Input: part model. Units: mm. Frame: model coordinates. A direction names the side the tool comes from. Coordinates: 2 decimals unless noted, no trailing zeros. Write each loop counter-clockwise with the first axis right and the second up, starting at its lowest first coordinate (ties: lowest second). Pieces come first, ordered by that corner, then holes. Notation, with made-up numbers: M 73.25,69 L 114.25,69 A19 ccw 114.25,93 Z; hole C 25.5,-19.75 d6. An arc over 180 degrees is marked long. Write each question's results on one line, items separated by ' | '. Start each with the question number.
1. First-contact query: pin 1 (6.5 mm diameter, centred on x = -12.06, z = -5, fed in from +Y); pin 2 (3 mm diameter, centred on x = -12.06, z = -25, fed in from +Y); pin 3 (10 mm diameter, centred on x = -13, z = -14, fed in from +Y). Flat tips, straight axial feed; report the tip coordinate or a pass-through.
2. Section query B-B, the plane x = 0. Output: boundary loops of the cut face in (y, z).
3. Section query C-C, the plane y = 0. Output: boundary loops of the cut face in (x, z).
4. Pull-direction query (X, two-part tool) for faces 4 (the flat face through (16.961, -2, -15)), 5 (the flat face through (4, -5, -30)), 6 (the cylindrical face through (-1.08, -4.88, -14.79)); classes: +X half, -X half, draft (parallel to the pull), parting line (faces both ways), or undercut.
5. Set-up query: faces 1 (the flat face through (-13, 7.001, -15)), 2 (the flat face through (12, 7.001, -15)), 3 (the flat face through (0, 11.001, -15)). Return all of +Z, -Z, +X, -X, +Y, -Y with unobstructed straight access to the full face (end or side cutting, diameter ignored); none if empty.
6. Section query A-A, the plane z = -5. Output: boundary loops of the cut face in (x, y), and give its area (3 significant figures).
7. Ray query, probe 1 along X at (y, z) = (1.5, -26.25); probe 2 along Z at (x, y) = (11, 6.5); probe 3 along Y at (x, z) = (0, -13.25). Return the intervals inside material, ascending.
8. Section query D-D, the plane x = 10.5. Output: boundary loops of the cut face in (y, z).
```python
from build123d import *

# Parameters (mm, degrees)
BOSS_EXTRUDE2_DEPTH    = 30
HOLE_R                 = 5
CUT_EXTRUDE1_DEPTH     = 30
CUT_EXTRUDE2_START     = -10.999447078
CUT_EXTRUDE2_OUTLINE_R = 2
CUT_EXTRUDE2_DEPTH     = 17.999956595


# Read off the part's stored shape, not the designer's step: Cut-Extrude2
with BuildPart() as part:
    # body → Boss-Extrude2 (new body)
    with BuildSketch(Plane.XY):
        Polygon((-8.038514806, 7.000509517), (-5.875565247, 11.000552922), (5.877594601, 11.000552922), (8.04054416, 7.000509517), (16.961485195, 7.000509517), (16.961485195, -10.999447078), (-17.038514805, -10.999447078), (-17.038514805, 7.000509517), align=None)
    extrude(amount=-BOSS_EXTRUDE2_DEPTH)

    # hole → Cut-Extrude1 (cut)
    with BuildSketch(Plane.XY):
        Circle(HOLE_R)
    extrude(amount=-CUT_EXTRUDE1_DEPTH, mode=Mode.SUBTRACT)

    # Cut-Extrude2 outline → Cut-Extrude2 (cut)
    with BuildSketch(Plane(origin=(0, 0, 0), x_dir=(1, 0, 0), z_dir=(0, 1, 0)).offset(CUT_EXTRUDE2_START)):
        with Locations((-12.061902792, 5)):
            Circle(CUT_EXTRUDE2_OUTLINE_R)
        with Locations((-12.061902792, 24.999986325)):
            Circle(CUT_EXTRUDE2_OUTLINE_R)
        with Locations((11.938097208, 24.999986325)):
            Circle(CUT_EXTRUDE2_OUTLINE_R)
        with Locations((11.938097208, 5)):
            Circle(CUT_EXTRUDE2_OUTLINE_R)
    extrude(amount=CUT_EXTRUDE2_DEPTH, mode=Mode.SUBTRACT)


solid = part.part
```
Answer:
1) pin 1: y = 7 | pin 2: through | pin 3: y = 7.07
2) outline: M -11,-30 L -5,-30 L -5,0 L -11,0 Z; M 5,-30 L 11,-30 L 11,0 L 5,0 Z
3) outline: M -17.04,-30 L -5,-30 L -5,0 L -17.04,0 Z; M 5,-30 L 16.96,-30 L 16.96,0 L 5,0 Z; hole C -12.06,-25 d4; hole C -12.06,-5 d4; hole C 11.94,-25 d4; hole C 11.94,-5 d4
4) face 4: +X half | face 5: draft | face 6: undercut
5) face 1: +Z, -Z, -X, +Y | face 2: +Z, -Z, +X, +Y | face 3: +Z, -Z, +X, -X, +Y
6) outline: M -17.04,-11 L -14.06,-11 L -14.06,7 L -17.04,7 Z; M -10.06,-11 L 9.94,-11 L 9.94,7 L 8.04,7 L 5.88,11 L -5.88,11 L -8.04,7 L -10.06,7 Z; M 13.94,-11 L 16.96,-11 L 16.96,7 L 13.94,7 Z; hole C 0,0 d10 | area: 445 mm^2
7) probe 1: -17.04 to -13.62, -10.5 to -4.77, 4.77 to 10.38, 13.5 to 16.96 | probe 2: -30 to -26.77, -23.23 to -6.77, -3.23 to 0 | probe 3: -11 to -5, 5 to 11
8) outline: M -11,-30 L 7,-30 L 7,-26.39 L -11,-26.39 Z; M -11,-23.61 L 7,-23.61 L 7,-6.39 L -11,-6.39 Z; M -11,-3.61 L 7,-3.61 L 7,0 L -11,0 Z
